from build123d import *

# Parameters (mm, degrees)
SKETCH1_W          = 76.2
SKETCH1_H          = 76.2
SKETCH1_W_2        = 57.15
SKETCH1_H_2        = 57.15
EXTRUDE1_DEPTH     = 107.95
SKETCH2_R          = 12.7
CUT_EXTRUDE1_DEPTH = 138.518189706
SKETCH3_R          = 12.7
CUT_EXTRUDE2_DEPTH = 138.518189706
SKETCH4_R          = 12.7
EXTRUDE2_DEPTH     = 12.7
SKETCH5_R          = 12.7
EXTRUDE3_DEPTH     = 12.7
FILLET1_R          = 9.525
FILLET2_R          = 3.175


with BuildPart() as part:
    # Sketch1 → Extrude1 (new, symmetric)
    with BuildSketch(Plane.XY):
        Rectangle(SKETCH1_W, SKETCH1_H)
        Rectangle(SKETCH1_W_2, SKETCH1_H_2, mode=Mode.SUBTRACT)
    extrude(amount=EXTRUDE1_DEPTH, both=True)

    # Sketch2 → Cut-Extrude1 (cut, through all)
    with BuildSketch(Plane(origin=(0, 38.1, 0), x_dir=(-1, 0, 0), z_dir=(0, 1, 0))):
        with Locations((0, 76.2)):
            Circle(SKETCH2_R)
    extrude(amount=-CUT_EXTRUDE1_DEPTH, mode=Mode.SUBTRACT)

    # Sketch3 → Cut-Extrude2 (cut, through all)
    with BuildSketch(Plane.ZY.offset(38.1)):
        with Locations(Location((-76.2, 0, 0), (0, 0, 270))):
            Circle(SKETCH3_R)
    extrude(amount=-CUT_EXTRUDE2_DEPTH, mode=Mode.SUBTRACT)

    # Sketch4 → Extrude2 (add, symmetric)
    with BuildSketch(Plane(origin=(0, 0, 0), x_dir=(0, 0, -1), z_dir=(1, 0, 0))):
        Polygon((-12.7, 38.1), (107.95, 38.1), (107.95, 63.5), (60.325, 101.6), (60.325, 190.5), (-12.7, 190.5), align=None)
        with Locations((31.75, 161.925)):
            Circle(SKETCH4_R, mode=Mode.SUBTRACT)
    extrude(amount=EXTRUDE2_DEPTH, both=True)

    # Sketch5 → Extrude3 (add, symmetric)
    with BuildSketch(Plane(origin=(0, 0, 0), x_dir=(1, 0, 0), z_dir=(0, 1, 0))):
        Polygon((38.1, 12.7), (38.1, -107.95), (63.5, -107.95), (101.6, -60.325), (190.5, -60.325), (190.5, 12.7), align=None)
        with Locations(Location((161.925, -31.75, 0), (0, 0, 270))):
            Circle(SKETCH5_R, mode=Mode.SUBTRACT)
    extrude(amount=EXTRUDE3_DEPTH, both=True)

    # Fillet1
    fillet1_edges = [part.edges().sort_by_distance(p)[0] for p in [
        (12.7, 38.1, -47.625),
        (-12.7, 38.1, -47.625),
        (0, 38.1, 12.7),
        (38.1, 12.7, 47.625),
        (38.1, -12.7, 47.625),
        (38.1, 0, -12.7),
    ]]
    fillet(fillet1_edges, radius=FILLET1_R)

    # Fillet2
    fillet2_edges = [part.edges().sort_by_distance(p)[0] for p in [
        (-28.575, 28.575, 0),
        (-28.575, -28.575, 0),
        (28.575, -28.575, 0),
        (28.575, 28.575, 0),
        (-38.1, 38.1, 0),
        (38.1, 38.1, 0),
        (38.1, -38.1, 0),
        (-38.1, -38.1, 0),
    ]]
    fillet(fillet2_edges, radius=FILLET2_R)


solid = part.part
The model under review builds one solid part; all positions refer to its coordinate system, in mm. A direction names the side the tool comes from. Round coordinates to 2 decimals unless told otherwise and drop trailing zeros. Write each loop counter-clockwise with the first axis right and the second up, starting at its lowest first coordinate (ties: lowest second). Pieces come first, ordered by that corner, then holes. Notation, with made-up numbers: M 88.5,9 L 111.5,9 A22 cw 111.5,25 Z; hole C 60.5,-15.75 d5. An arc over 180 degrees is marked long. Use a Markdown table: item, result. Add a question column.
Q1. We need section D-D, the plane y = 0. State the section outline as (x, z) points (3 decimals), plus the area to 3 significant figures.
Q2. To check wall thickness, follow line 1 (Y direction, x = 0.25, z = -31.75) (3 decimals); line 2 (X direction, y = 12, z = 47) (3 decimals). State the ranges of each line that lie inside material, in increasing order.
Q3. We need section A-A, the plane z = 29. State the section outline as (x, y) points (3 decimals), plus the area to 3 significant figures.
Q4. Insertion check: pin 1 (4 mm diameter, centred on y = 22.5, z = 59, fed in from +X); pin 2 (20.5 mm diameter, centred on x = -4.5, y = 148.5, fed in from -Z) (3 decimals); pin 3 (7.5 mm diameter, centred on x = 137.5, y = 1, fed in from +Z) (3 decimals). Each pin has a flat end and moves straight along its axis. Give the tip position at first contact, or say it passes through.
Q5. We need section C-C, the plane z = -57. State the section outline as (x, y) points (3 decimals), plus the area to 3 significant figures.
Q6. We need section B-B, the plane x = 0. State the section outline as (y, z) points (3 decimals).
Q7. The part is to be moulded in two halves that separate along Y. For faces 6 (the face through (0, 28.575, 2)), 7 (the face through (33.271, -12.114, -72.385)), 8 (the face through (40.82, -15.56, 43.77)), 9 (the face through (0, 120, 12.7)), say which applies: pulls with the +Y half, pulls with the -Y half, needs draft (parallel to the pull), parting line crosses it, or undercut.
Q8. Machinability: for faces 1 (the face through (-28.575, 0, 2)), 2 (the face through (118, 12.7, 33)), 3 (the face through (0, 145, -60.325)), 4 (the face through (0, 38.1, 26)), 5 (the face through (118, -12.7, 33)), which of the approach directions +Z, -Z, +X, -X, +Y, -Y give a long, thin tool a straight path to every point of the face, cutting with its end or side? Answer none if there is none.
Findings below:
| question | item | result |
|---|---|---|
| 1 | outline | M -38.1,-107.95 L -28.575,-107.95 L -28.575,-88.9 L -38.1,-88.9 Z; M -38.1,-63.5 L -28.575,-63.5 L -28.575,107.95 L -38.1,107.95 Z; M 28.575,-107.95 L 38.1,-107.95 L 38.1,-88.9 L 28.575,-88.9 Z; M 28.575,-63.5 L 38.1,-63.5 L 38.1,-22.225 A9.525 cw 47.625,-12.7 L 190.5,-12.7 L 190.5,60.325 L 101.6,60.325 L 63.5,107.95 L 28.575,107.95 Z; hole C 161.925,31.75 d25.4 |
| 1 | area | 16,400 mm² |
| 2 | line 1 | y = -38.1 to -28.575, 28.575 to 149.225, 174.625 to 190.5 |
| 2 | line 2 | x = -38.1 to -28.575, 28.575 to 190.5 |
| 3 | outline | M -38.1,-34.925 A3.175 ccw -34.925,-38.1 L 34.925,-38.1 A3.175 ccw 38.1,-34.925 L 38.1,-22.225 A9.525 cw 47.625,-12.7 L 149.526,-12.7 L 149.526,12.7 L 47.625,12.7 A9.525 cw 38.1,22.225 L 38.1,34.925 A3.175 ccw 34.925,38.1 L -34.925,38.1 A3.175 ccw -38.1,34.925 Z; M 174.324,-12.7 L 190.5,-12.7 L 190.5,12.7 L 174.324,12.7 Z; hole M -28.575,-25.4 A3.175 ccw -25.4,-28.575 L 25.4,-28.575 A3.175 ccw 28.575,-25.4 L 28.575,25.4 A3.175 ccw 25.4,28.575 L -25.4,28.575 A3.175 ccw -28.575,25.4 Z |
| 3 | area | 5,820 mm² |
| 4 | pin 1 | stops at x = 38.26 |
| 4 | pin 2 | stops at z = -60.325 |
| 4 | pin 3 | stops at z = 60.325 |
| 5 | outline | M -38.1,-34.925 A3.175 ccw -34.925,-38.1 L 34.925,-38.1 A3.175 ccw 38.1,-34.925 L 38.1,34.925 A3.175 ccw 34.925,38.1 L 22.225,38.1 A9.525 cw 12.7,47.625 L 12.7,190.5 L -12.7,190.5 L -12.7,47.625 A9.525 cw -22.225,38.1 L -34.925,38.1 A3.175 ccw -38.1,34.925 Z; hole M -28.575,-25.4 A3.175 ccw -25.4,-28.575 L 25.4,-28.575 A3.175 ccw 28.575,-25.4 L 28.575,25.4 A3.175 ccw 25.4,28.575 L -25.4,28.575 A3.175 ccw -28.575,25.4 Z |
| 5 | area | 6,450 mm² |
| 6 | outline | M -38.1,-107.95 L -28.575,-107.95 L -28.575,63.5 L -38.1,63.5 Z; M -38.1,88.9 L -28.575,88.9 L -28.575,107.95 L -38.1,107.95 Z; M 28.575,-107.95 L 63.5,-107.95 L 101.6,-60.325 L 190.5,-60.325 L 190.5,12.7 L 47.625,12.7 A9.525 cw 38.1,22.225 L 38.1,63.5 L 28.575,63.5 Z; M 28.575,88.9 L 38.1,88.9 L 38.1,107.95 L 28.575,107.95 Z; hole C 161.925,-31.75 d25.4 |
| 7 | face 6 | undercut |
| 7 | face 7 | undercut |
| 7 | face 8 | pulls with the -Y half |
| 7 | face 9 | needs draft |
| 8 | face 1 | +Z, -Z |
| 8 | face 2 | +Z, -Z, +X, +Y |
| 8 | face 3 | -Z, +X, -X, +Y |
| 8 | face 4 | +Z, +Y |
| 8 | face 5 | +Z, -Z, +X, -Y |
